Geometry: final body of the model. Coordinates: model frame, mm. A direction names the side the tool comes from. Give positions to 0.01 mm unless a question says otherwise; leave off trailing zeros. Loops run counter-clockwise (first coordinate to the right, second up) from the corner with the lowest first, then second, coordinate; pieces in that order, holes last.
1. Draft query along Y for faces 1 (the face through (10, 5, 0)), 2 (the face through (4.38, -8.43, 12.07)). Return one class per face: +Y half, -Y half, draft (parallel to the pull), parting line (faces both ways), or undercut.
2. First-contact query: P1, Ø20, axis at x = 0, y = 0, coming from the -Z side; P2, Ø3, axis at y = -24, z = 17.5, coming from the -X side; P3, Ø17.5, axis at x = 0, y = 0, coming from the -Z side; P4, Ø10, axis at y = 14, z = 4, coming from the -X side. Flat tips, straight axial feed; report the tip coordinate or a pass-through.
3. Section D-D, the plane z = 9. Output: boundary loops of the cut face in (x, y), then the cut area to 3 significant figures.
4. Material intervals for line 1 along Y through (x, z) = (-7.5, 20.25); line 2 along X through (y, z) = (4, 2.5); line 3 along Y through (x, z) = (-2.5, 18.75), sorted ascending.
5. Access query for faces 3 (the face through (-2.38, 10.74, 3.55)), 4 (the face through (10, 5, 24)), 5 (the face through (-2.38, -10.74, 20.55)). Directions: +Z, -Z, +X, -X, +Y, -Y. A direction counts if a zero-diameter tool reaches every point of the face in a straight line with its end or side. Return the directions, or none.
6. Section C-C, the plane z = 18. Output: boundary loops of the cut face in (x, y).
from build123d import *

# Parameters (mm, degrees)
ESQUISSE1_R             = 35
EXTRUSION1_DEPTH        = 24
CONG_1_R                = 12
CONG_2_R                = 12
ESQUISSE2_R             = 11
ENL_V_MAT_EXTRU_1_DEPTH = 7
ENL_V_START             = -7
ESQUISSE3_R             = 11
ENL_V_MAT_EXTRU_2_DEPTH = 7
ESQUISSE5_R             = 9.5
ENL_V_MAT_EXTRU_3_DEPTH = 53.335456499


with BuildPart() as part:
    # Esquisse1 → Extrusion1 (new body)
    with BuildSketch(Plane.XY):
        Circle(ESQUISSE1_R)
    extrude(amount=EXTRUSION1_DEPTH)

    # Congé1
    cong_1_edges = [part.edges().sort_by_distance(p)[0] for p in [
        (-35, 0, 24),
    ]]
    fillet(cong_1_edges, radius=CONG_1_R)

    # Congé2
    cong_2_edges = [part.edges().sort_by_distance(p)[0] for p in [
        (-35, 0, 0),
    ]]
    fillet(cong_2_edges, radius=CONG_2_R - 0.0001)  # a hair under: the kernel refuses the full size

    # Esquisse2 → Enlèv. mat.-Extru.1 (cut)
    with BuildSketch(Plane.XY.offset(24)):
        Circle(ESQUISSE2_R)
    extrude(amount=-ENL_V_MAT_EXTRU_1_DEPTH, mode=Mode.SUBTRACT)

    # Esquisse3 → Enlèv. mat.-Extru.2 (cut)
    with BuildSketch(Plane(origin=(0, 0, 0), x_dir=(-1, 0, 0), z_dir=(0, 0, -1)).offset(ENL_V_START)):
        with Locations(Location((0, 0, 0), (0, 0, 180))):
            Circle(ESQUISSE3_R)
    extrude(amount=ENL_V_MAT_EXTRU_2_DEPTH, mode=Mode.SUBTRACT)

    # Esquisse5 → Enlèv. mat.-Extru.3 (cut, through all)
    with BuildSketch(Plane.XY.offset(17)):
        Circle(ESQUISSE5_R)
    extrude(amount=-ENL_V_MAT_EXTRU_3_DEPTH, mode=Mode.SUBTRACT)


solid = part.part
Answers below:
1. face 1: draft
1. face 2: undercut
2. P1: stops at z = 7
2. P2: stops at x = -25.34
2. P3: passes through
2. P4: stops at x = -32.51
3. outline: circle Ø69.24 at (0, 0); hole circle Ø19 at (0, 0)
3. area: 3,480 mm2
4. line 1: y = -30.81 to -8.05, 8.05 to 30.81
4. line 2: x = -30.07 to -10.25, 10.25 to 30.07
4. line 3: y = -32.83 to -10.71, 10.71 to 32.83
5. face 3: -Z
5. face 4: +Z, +X, -X, +Y, -Y
5. face 5: +Z
6. outline: circle Ø66.78 at (0, 0); hole circle Ø22 at (0, 0)
